```python
from build123d import *

# Parameters (mm, degrees)
SKETCH1_R                   = 48.5
SKETCH1_R_2                 = 2.75
BOSS_EXTRUDE1_DEPTH         = 5
F_1_4_0_25_DIAMETER_HOLE1_D = 6.35
FILLET1_R                   = 5


with BuildPart() as part:
    # Sketch1 → Boss-Extrude1 (new body, symmetric)
    with BuildSketch(Plane(origin=(0, 0, 0), x_dir=(1, 0, 0), z_dir=(0, 1, 0))):
        with BuildLine():
            Line((-102.265318229, 19.53382483), (-41.365746699, -41.365746699))
            ThreePointArc((-41.365746699, -41.365746699), (8.808484383, -57.833040754), (51.805109545, -27.175))
            Line((51.805109545, -27.175), (79.375, -27.175))
            Line((79.375, -27.175), (79.375, 27.175))
            Line((79.375, 27.175), (51.805109545, 27.175))
            ThreePointArc((51.805109545, 27.175), (30.269724974, 50.059901618), (0, 58.5))
            Line((0, 58.5), (-122.342559288, 58.5))
            Line((-122.342559288, 58.5), (-131.787026344, 49.055532945))
            Line((-131.787026344, 49.055532945), (-102.265318229, 19.53382483))
        make_face()
        Circle(SKETCH1_R, mode=Mode.SUBTRACT)
        with Locations((-123.832075055, 48.87875625)):
            Circle(SKETCH1_R_2, mode=Mode.SUBTRACT)
        with Locations((-98.376230933, 23.422912127)):
            Circle(SKETCH1_R_2, mode=Mode.SUBTRACT)
        with Locations((53.5, 18)):
            Circle(SKETCH1_R_2, mode=Mode.SUBTRACT)
        with Locations((53.5, -18)):
            Circle(SKETCH1_R_2, mode=Mode.SUBTRACT)
        with BuildLine():
            Line((-88.123182605, 19.53382483), (-57.4247459, -11.164611875))
            ThreePointArc((-57.4247459, -11.164611875), (-54.046952652, 22.386980793), (-32.710854468, 48.5))
            Line((-32.710854468, 48.5), (-59.157007436, 48.5))
            Line((-59.157007436, 48.5), (-88.123182605, 19.53382483))
        make_face(mode=Mode.SUBTRACT)
    extrude(amount=BOSS_EXTRUDE1_DEPTH, both=True)

    # 1/4 (0.25) Diameter Hole1 (through all)
    with Locations(Plane(origin=(0, 5, 0), x_dir=(1, 0, 0), z_dir=(0, 1, 0))):
        with Locations((71.2, 19), (71.2, 0), (71.2, -19)):
            Hole(F_1_4_0_25_DIAMETER_HOLE1_D / 2)

    # Fillet1
    fillet1_edges = [part.edges().sort_by_distance(p)[0] for p in [
        (-122.342559288, 0, -58.5),
        (51.805109545, 0, -27.175),
        (79.375, 0, -27.175),
        (79.375, 0, 27.175),
        (51.805109545, 0, 27.175),
        (-88.123182605, 0, -19.53382483),
        (-59.157007436, 0, -48.5),
        (-32.710854468, 0, -48.5),
        (-57.4247459, 0, 11.164611875),
    ]]
    fillet(fillet1_edges, radius=FILLET1_R)


solid = part.part
```
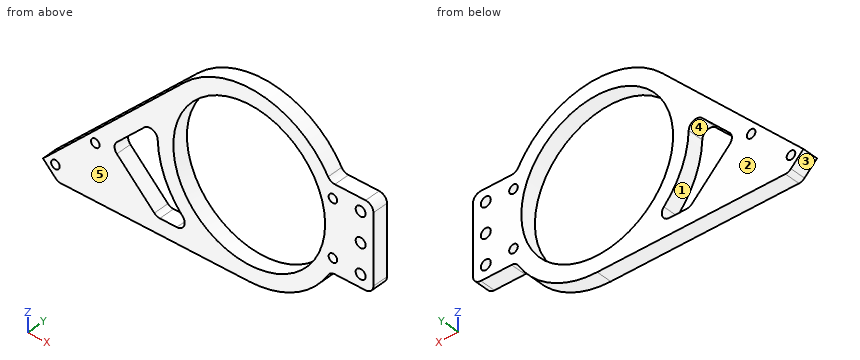
Here's how the part is built. I have some questions about the finished solid (model axes, mm). Face numbers are marked on the shaded views. A direction names the side the tool comes from. Coordinates: 2 decimals unless noted, no trailing zeros. Order: outer loops, then holes, each group sorted by start corner. A loop starts at its lowest first (then second) coordinate and runs counter-clockwise, first axis right, second up.
Item 1: If we section it at D-D, the plane z = -34: List the corners of the cut face in (x, y) for me.
Response values:
outline: (-116.73, -5) - (-73.66, -5) - (-73.66, 5) - (-116.73, 5) - close; (-47.61, -5) - (-34.59, -5) - (-34.59, 5) - (-47.61, 5) - close; (34.59, -5) - (47.61, -5) - (47.61, 5) - (34.59, 5) - close
Item 2: Thinking about a two-plate mould opening in X: for the marked faces 1, 2 and 3, which applies, pulls with the +X half, pulls with the -X half, needs draft (parallel to the pull), parting line crosses it, or undercut?
Response values:
face 1: undercut
face 2: needs draft
face 3: pulls with the -X half
Item 3: Which directions (+Z, -Z, +X, -X, +Y, -Y) give clear straight access to the entire face, cutting with the end or side of a thin tool? Please do the marked faces 4 and 5.
Response values:
face 4: +Y, -Y
face 5: +Z, -Z, +X, -X, -Y
Item 4: If we section it at B-B, the plane z = 34: List the corners of the cut face in (x, y) for me, then the cut area to 3 significant figures.
Response values:
outline: (-48.73, -5) - (-34.59, -5) - (-34.59, 5) - (-48.73, 5) - close; (34.59, -5) - (47.61, -5) - (47.61, 5) - (34.59, 5) - close
area: 272 mm2
Item 5: I need wall thicknesses on probe 1 along Z at (x, y) = (71.2, 0.5) (3 decimals); probe 2 along X at (y, z) = (-3, -1.5) (1 decimal); probe 3 along Z at (x, y) = (-43, 0.5). Which ranges of each line are inside material? Lowest first, please.
Response values:
probe 1: z = -27.175 to -22.175, -15.825 to -3.175, 3.175 to 15.825, 22.175 to 27.175
probe 2: x = -84.2 to -70.1, -58.5 to -48.5, 48.5 to 68.4, 74 to 79.4
probe 3: z = -58.5 to -47.29, -39.66 to -22.43, 22.43 to 39.73
Item 6: I'm going to push flat-ended pins straight in: pin 1 Ø3 at (x, y) = (61, -2.5) entering from -Z (3 decimals); pin 2 Ø3 at (x, y) = (-53.5, 0) entering from +Z; pin 3 Ø4 at (y, z) = (-0.5, 16.5) entering from -X; pin 4 Ø5 at (x, z) = (71.2, 0) entering from +Y. Where does each tip first touch, or does it pass through?
Response values:
pin 1: stops at z = -27.175
pin 2: stops at z = 30.73
pin 3: stops at x = -68.23
pin 4: passes through
Item 7: If we section it at C-C, the plane y = 2.5: Give the number of separate pieces and of enclosed holes in the cut face, then the cut area to 3 significant figures.
Response values:
separate pieces: 1
enclosed holes: 9
area: 7,380 mm2
Item 8: If we section it at A-A, the plane x = 40.5: List the corners of the cut face in (y, z) for me, then the cut area to 3 significant figures.
Response values:
outline: (-5, -42.21) - (5, -42.21) - (5, -26.68) - (-5, -26.68) - close; (-5, 26.68) - (5, 26.68) - (5, 42.21) - (-5, 42.21) - close
area: 311 mm2
